Can you work these out from the model? Positions are in its coordinate system, mm. Round coordinates to 2 decimals unless told otherwise and drop trailing zeros. Order: outer loops, then holes, each group sorted by start corner. A loop starts at its lowest first (then second) coordinate and runs counter-clockwise, first axis right, second up. Notation, with made-up numbers: M -10,33.5 L 32,33.5 A20 ccw 32,71.5 Z; hole C -34.5,28 d8. An arc over 180 degrees is marked long. Answer as a JSON object with one key per item and string values. Group by question number.
```python
from build123d import *

# Parameters (mm, degrees)
SKETCH_R   = 11.75
SKETCH_R_2 = 1.8288
PAD_DEPTH  = 3


with BuildPart() as part:
    # Sketch → Pad (new body)
    with BuildSketch(Plane.XY):
        with BuildLine():
            ThreePointArc((-78.2, 50.8), (-78.907107, 50.507107), (-79.2, 49.8))
            Line((-79.2, -49.8), (-79.2, 49.8))
            ThreePointArc((-79.2, -49.8), (-78.907107, -50.507107), (-78.2, -50.8))
            Line((-78.2, -50.8), (-35.877, -50.8))
            ThreePointArc((-35.877, -50.8), (-35.169893, -50.507107), (-34.877, -49.8))
            Line((-34.877, -38.1), (-34.877, -49.8))
            ThreePointArc((-28.273, -38.1), (-31.575, -34.798), (-34.877, -38.1))
            Line((-28.273, -38.1), (-28.273, -49.8))
            ThreePointArc((-28.273, -49.8), (-27.980107, -50.507107), (-27.273, -50.8))
            Line((-27.273, -50.8), (27.273, -50.8))
            ThreePointArc((27.273, -50.8), (27.980107, -50.507107), (28.273, -49.8))
            Line((28.273, -38.1), (28.273, -49.8))
            ThreePointArc((34.877, -38.1), (31.575, -34.798), (28.273, -38.1))
            Line((34.877, -38.1), (34.877, -49.8))
            ThreePointArc((34.877, -49.8), (35.169893, -50.507107), (35.877, -50.8))
            Line((35.877, -50.8), (78.2, -50.8))
            ThreePointArc((78.2, -50.8), (78.907107, -50.507107), (79.2, -49.8))
            Line((79.2, 49.8), (79.2, -49.8))
            ThreePointArc((79.2, 49.8), (78.907107, 50.507107), (78.2, 50.8))
            Line((-78.2, 50.8), (78.2, 50.8))
        make_face()
        with Locations((0, -3.175)):
            Circle(SKETCH_R, mode=Mode.SUBTRACT)
        with Locations((-65.7352, 44.45)):
            Circle(SKETCH_R_2, mode=Mode.SUBTRACT)
        with Locations((65.7352, 44.45)):
            Circle(SKETCH_R_2, mode=Mode.SUBTRACT)
        with BuildLine():
            ThreePointArc((-13.3, 21.825), (-13.441421, 21.766421), (-13.5, 21.625))
            Line((-13.5, 18.025), (-13.5, 21.625))
            ThreePointArc((-13.5, 18.025), (-13.441421, 17.883579), (-13.3, 17.825))
            Line((-11.7, 17.825), (-13.3, 17.825))
            ThreePointArc((-11.7, 17.825), (-11.558579, 17.883579), (-11.5, 18.025))
            Line((-11.5, 21.625), (-11.5, 18.025))
            ThreePointArc((-11.5, 21.625), (-11.558579, 21.766421), (-11.7, 21.825))
            Line((-13.3, 21.825), (-11.7, 21.825))
        make_face(mode=Mode.SUBTRACT)
        with BuildLine():
            ThreePointArc((11.7, 21.825), (11.558579, 21.766421), (11.5, 21.625))
            Line((11.5, 18.025), (11.5, 21.625))
            ThreePointArc((11.5, 18.025), (11.558579, 17.883579), (11.7, 17.825))
            Line((13.3, 17.825), (11.7, 17.825))
            ThreePointArc((13.3, 17.825), (13.441421, 17.883579), (13.5, 18.025))
            Line((13.5, 21.625), (13.5, 18.025))
            ThreePointArc((13.5, 21.625), (13.441421, 21.766421), (13.3, 21.825))
            Line((11.7, 21.825), (13.3, 21.825))
        make_face(mode=Mode.SUBTRACT)
    extrude(amount=PAD_DEPTH)


solid = part.part
```
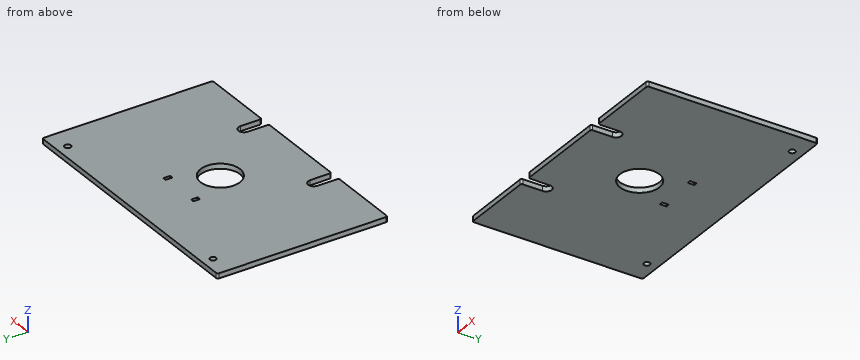
1) If we section it at A-A on x = 0: Write out the boundary of the cut face in (y, z) (3 decimals).
2) If we section it at D-D on x = 31: Write out the boundary of the cut face in (y, z), plus the area to 3 significant figures.
3) If we section it at C-C on y = -1: Write out the boundary of the cut face in (x, z).
4) If we section it at B-B on y = 44.45: Write out the boundary of the cut face in (x, z).
5) I need wall thicknesses on line 1 along X through (y, z) = (-44.5, 1.4); line 2 along Y through (x, z) = (0, 1) (3 decimals); line 3 along X through (y, z) = (7, 1.15). Which ranges of each line are inside material? Lowest first, please.
Findings:
{
 "1": {"outline": "M -50.8,0 L -14.925,0 L -14.925,3 L -50.8,3 Z; M 8.575,0 L 50.8,0 L 50.8,3 L 8.575,3 Z"},
 "2": {"outline": "M -34.85,0 L 50.8,0 L 50.8,3 L -34.85,3 Z", "area": "257 mm^2"},
 "3": {"outline": "M -79.2,0 L -11.55,0 L -11.55,3 L -79.2,3 Z; M 11.55,0 L 79.2,0 L 79.2,3 L 11.55,3 Z"},
 "4": {"outline": "M -79.2,0 L -67.56,0 L -67.56,3 L -79.2,3 Z; M -63.91,0 L 63.91,0 L 63.91,3 L -63.91,3 Z; M 67.56,0 L 79.2,0 L 79.2,3 L 67.56,3 Z"},
 "5": {"line 1": "x = -79.2 to -34.88, -28.27 to 28.27, 34.88 to 79.2", "line 2": "y = -50.8 to -14.925, 8.575 to 50.8", "line 3": "x = -79.2 to -5.88, 5.88 to 79.2"}
}
